```python
from build123d import *

# Parameters (mm, degrees)
SKETCH1_R           = 7.5
DISK1_DEPTH         = 5
SKETCH2_R           = 7.5
DISK2_DEPTH         = 5
SKETCH3_R           = 7
TAP_GAP_DEPTH       = 1
SKETCH4_R           = 6
TOP_BEARING_DEPTH   = 5
SHAFTMOUNT_R        = 7
GAP_DEPTH           = 1
SKETCH8_R           = 6
BEARING_DEPTH       = 5
SKETCH9_R           = 6
SKETCH9_R_2         = 5
BOSS_EXTRUDE2_DEPTH = 5
SKETCH7_R           = 2.75
HOLECUT_DEPTH       = 20.397164741
HOLECUT_DEPTH_BACK  = 20.397164741


with BuildPart() as part:
    # Sketch1 → disk1 (new body)
    with BuildSketch(Plane(origin=(0, 0, 0), x_dir=(1, 0, 0), z_dir=(0, 1, 0))):
        with Locations(Location((-0.5, 0, 0), (0, 0, 270))):
            Circle(SKETCH1_R)
    extrude(amount=DISK1_DEPTH)

    # Sketch2 → disk2 (add)
    with BuildSketch(Plane(origin=(0, 5, 0), x_dir=(1, 0, 0), z_dir=(0, 1, 0))):
        with Locations(Location((0.5, 0, 0), (0, 0, 93.822553729))):
            Circle(SKETCH2_R)
    extrude(amount=DISK2_DEPTH)

    # Sketch3 → tap-gap (add)
    with BuildSketch(Plane(origin=(0, 10, 0), x_dir=(1, 0, 0), z_dir=(0, 1, 0))):
        with Locations(Location((0, 0, 0), (0, 0, 180))):
            Circle(SKETCH3_R)
    extrude(amount=TAP_GAP_DEPTH)

    # Sketch4 → top-bearing (add)
    with BuildSketch(Plane(origin=(0, 11, 0), x_dir=(1, 0, 0), z_dir=(0, 1, 0))):
        with Locations(Location((0, 0, 0), (0, 0, 270))):
            Circle(SKETCH4_R)
    extrude(amount=TOP_BEARING_DEPTH)

    # shaftmount → gap (add)
    with BuildSketch(Plane(origin=(0, 0, 0), x_dir=(1, 0, 0), z_dir=(0, 1, 0))):
        with Locations(Location((0, 0, 0), (0, 0, 180))):
            Circle(SHAFTMOUNT_R)
    extrude(amount=-GAP_DEPTH)

    # Sketch8 → bearing (add)
    with BuildSketch(Plane.XZ.offset(1)):
        with Locations(Location((0, 0, 0), (0, 0, 90))):
            Circle(SKETCH8_R)
    extrude(amount=BEARING_DEPTH)

    # Sketch9 → Boss-Extrude2 (add)
    with BuildSketch(Plane.XZ.offset(6)):
        with Locations(Location((0, 0, 0), (0, 0, 90))):
            Circle(SKETCH9_R)
        Circle(SKETCH9_R_2, mode=Mode.SUBTRACT)
        with BuildLine():
            Line((-3, -4), (-3, 4))
            ThreePointArc((-3, 4), (-5, 0), (-3, -4))
        make_face()
    extrude(amount=BOSS_EXTRUDE2_DEPTH)

    # Sketch7 → holeCut (cut, two sides)
    with BuildSketch(Plane(origin=(0, 0, 0), x_dir=(1, 0, 0), z_dir=(0, 1, 0))) as holecut_sk:
        with Locations(Location((0, 0, 0), (0, 0, 270))):
            Circle(SKETCH7_R)
    extrude(amount=HOLECUT_DEPTH, mode=Mode.SUBTRACT)
    extrude(holecut_sk.sketch, amount=-HOLECUT_DEPTH_BACK, mode=Mode.SUBTRACT)


solid = part.part
```
Part model, mm, in its own coordinate system. A direction names the side the tool comes from. Round coordinates to 2 decimals unless told otherwise and drop trailing zeros. Loops run counter-clockwise (first coordinate to the right, second up) from the corner with the lowest first, then second, coordinate; pieces in that order, holes last.
Item 1: Cut at C-C, the plane y = -6.5. Give the cut face in (x, z), then the cut area to 3 significant figures.
Item 2: Drill centre lines: line 1 (X direction, y = 4.25, z = 0); line 2 (X direction, y = 6.25, z = 0); line 3 (Y direction, x = 4, z = -2.25). Where is each one in solid material? Low to high.
Item 3: Drop flat-ended pins along their axis: P1, Ø2.5, axis at y = -8, z = 0, coming from the +X side; P2, Ø3, axis at x = -3, y = -6.5, coming from the +Z side; P3, Ø1.5, axis at x = 6.5, z = -2, coming from the +Y side. Give the stop position or say it passes through.
Item 4: Mould opens along Z. For faces 1 (the face through (7.2, 10, 0.1)), 2 (the face through (3, -6, 1)), 3 (the face through (-6.466, -0.493, -2.681)) say: +Z half, -Z half, draft (parallel to the pull), parting line (faces both ways), or undercut.
Item 5: 3-axis set-ups, long thin cutter, end or side, ignore diameter. For faces 4 (the face through (7.2, 5, 0.1)), 5 (the face through (-7.2, 5, 0)), 6 (the face through (-6, -1, 2)), 7 (the face through (5, 7, 6)): which of +Z, -Z, +X, -X, +Y, -Y reach the whole face in a straight line?
Item 6: Cut at D-D, the plane x = 5.5. Give the cut face in (y, z), then the cut area to 3 significant figures.
A:
1. outline: circle Ø12 at (0, 0); hole (-3, -4) arc R5 ccw (long way) to (-3, 4) - close
1. area: 45.7 mm2
2. line 1: x = -8 to -2.75, 2.75 to 7
2. line 2: x = -7 to -2.75, 2.75 to 8
2. line 3: y = -6 to 16
3. P1: stops at x = 6
3. P2: stops at z = 5.81
3. P3: stops at y = 11
4. face 1: draft
4. face 2: undercut
4. face 3: parting line
5. face 4: +X, -Y
5. face 5: -X, +Y
5. face 6: -Y
5. face 7: +Y
6. outline: (-11, -2.4) - (-1, -2.4) - (-1, -4.33) - (0, -4.33) - (0, -4.5) - (5, -4.5) - (5, -5.59) - (10, -5.59) - (10, -4.33) - (11, -4.33) - (11, -2.4) - (16, -2.4) - (16, 2.4) - (11, 2.4) - (11, 4.33) - (10, 4.33) - (10, 5.59) - (5, 5.59) - (5, 4.5) - (0, 4.5) - (0, 4.33) - (-1, 4.33) - (-1, 2.4) - (-11, 2.4) - close
6. area: 190 mm2
